```python
from build123d import *

# Parameters (mm, degrees)
SKETCH1_W           = 138.0236
SKETCH1_H           = 34.1122
BOSS_EXTRUDE1_DEPTH = 145.034
SKETCH2_R           = 11.43
BOSS_EXTRUDE2_DEPTH = 15.24
SKETCH3_R           = 7.62
BOSS_EXTRUDE3_DEPTH = 3.81


with BuildPart() as part:
    # Sketch1 → Boss-Extrude1 (new body)
    with BuildSketch(Plane(origin=(0, 0, 0), x_dir=(1, 0, 0), z_dir=(0, 1, 0))):
        Rectangle(SKETCH1_W, SKETCH1_H)
    extrude(amount=BOSS_EXTRUDE1_DEPTH)

    # Sketch2 → Boss-Extrude2 (add)
    with BuildSketch(Plane(origin=(0, 145.034, 0), x_dir=(1, 0, 0), z_dir=(0, 1, 0))):
        with Locations((-35.4584, 0)):
            Circle(SKETCH2_R)
        with Locations((35.4584, 0)):
            Circle(SKETCH2_R)
    extrude(amount=BOSS_EXTRUDE2_DEPTH)

    # Sketch3 → Boss-Extrude3 (add)
    with BuildSketch(Plane(origin=(0, 145.034, 0), x_dir=(1, 0, 0), z_dir=(0, 1, 0))):
        Circle(SKETCH3_R)
    extrude(amount=BOSS_EXTRUDE3_DEPTH)


solid = part.part
```
Could you check a few things on this model? Use its own coordinates, in mm. A direction names the side the tool comes from. Give positions to 0.01 mm unless a question says otherwise; leave off trailing zeros. Loops run counter-clockwise (first coordinate to the right, second up) from the corner with the lowest first, then second, coordinate; pieces in that order, holes last. Notation, with made-up numbers: (2.5, 3) -> (48.5, 3) arc R22 cw to (48.5, 30) -> close; hole circle Ø5 at (53, 55). An arc over 180 degrees is marked (long way). Put each result on its own line as item: value.
(1) For faces 5 (the face through (0, 148.844, 0)), 6 (the face through (35, 160.274, 0)), 7 (the face through (-24.556, 152.547, -3.433)), which set-ups out of +Z, -Z, +X, -X, +Y, -Y let a thin tool reach every point of the face, with its end or its side?
Computed:
face 5: +Z, -Z, +Y
face 6: +Z, -Z, +X, -X, +Y
face 7: +Y
(2) Imagine slicing it at B-B on x = 0. Write out the boundary of the cut face in (y, z), plus the area to 3 significant figures.
Computed:
outline: (0, -17.06) -> (145.03, -17.06) -> (145.03, -7.62) -> (148.84, -7.62) -> (148.84, 7.62) -> (145.03, 7.62) -> (145.03, 17.06) -> (0, 17.06) -> close
area: 5,010 mm^2
(3) I'm going to push flat-ended pins straight in: pin 1 Ø4 at (x, z) = (8.5, 12) entering from +Y; pin 2 Ø7.5 at (x, z) = (3.5, 3) entering from +Y. Where does each tip first touch, or does it pass through?
Computed:
pin 1: y = 145.03
pin 2: y = 148.84
(4) Imagine slicing it at D-D on z = 9.5. Write out the boundary of the cut face in (x, y), plus the area to 3 significant figures.
Computed:
outline: (-69.01, 0) -> (69.01, 0) -> (69.01, 145.03) -> (41.81, 145.03) -> (41.81, 160.27) -> (29.1, 160.27) -> (29.1, 145.03) -> (-29.1, 145.03) -> (-29.1, 160.27) -> (-41.81, 160.27) -> (-41.81, 145.03) -> (-69.01, 145.03) -> close
area: 20,400 mm^2
(5) Imagine slicing it at C-C on x = 40. Write out the boundary of the cut face in (y, z), plus the area to 3 significant figures.
Computed:
outline: (0, -17.06) -> (145.03, -17.06) -> (145.03, -10.49) -> (160.27, -10.49) -> (160.27, 10.49) -> (145.03, 10.49) -> (145.03, 17.06) -> (0, 17.06) -> close
area: 5,270 mm^2
(6) Thinking about a two-plate mould opening in X: for faces 1 (the face through (-1, 145.034, -8)), 2 (the face through (-1, 72, -17.056)), 3 (the face through (-69.012, 72, 0)), 4 (the face through (69.012, 72, 0)), which applies, pulls with the +X half, pulls with the -X half, needs draft (parallel to the pull), parting line crosses it, or undercut?
Computed:
face 1: undercut
face 2: needs draft
face 3: pulls with the -X half
face 4: pulls with the +X half
(7) Imagine slicing it at A-A on z = 0. Write out the boundary of the cut face in (x, y), plus the area to 3 significant figures.
Computed:
outline: (-69.01, 0) -> (69.01, 0) -> (69.01, 145.03) -> (46.89, 145.03) -> (46.89, 160.27) -> (24.03, 160.27) -> (24.03, 145.03) -> (7.62, 145.03) -> (7.62, 148.84) -> (-7.62, 148.84) -> (-7.62, 145.03) -> (-24.03, 145.03) -> (-24.03, 160.27) -> (-46.89, 160.27) -> (-46.89, 145.03) -> (-69.01, 145.03) -> close
area: 20,800 mm^2
(8) Please list where these lines run through material, in increasing order: probe 1 along Y at (x, z) = (-56.5, -12.5); probe 2 along Z at (x, y) = (-32.5, 153). Write a range as [from, to].
Computed:
probe 1: [0, 145.03]
probe 2: [-11.04, 11.04]
